The listing builds one solid part. Answer for the finished solid, in the listing's coordinates (mm). A direction names the side the tool comes from. Coordinates: 2 decimals unless noted, no trailing zeros. Order: outer loops, then holes, each group sorted by start corner. A loop starts at its lowest first (then second) coordinate and runs counter-clockwise, first axis right, second up.
from build123d import *

# Parameters (mm, degrees)
SKETCH2_R                            = 3.35
F_40_SERIES_TS40_80LM_650037_1_DEPTH = 300
M8X1_25_TAPPED_HOLE1_AT_2_COUNT      = 2
M8X1_25_TAPPED_HOLE1_AT_2_PITCH      = 40


with BuildPart() as part:
    # Sketch2 → 40 series TS40-80LM-650037(1) (new body)
    with BuildSketch(Plane(origin=(0, 0, 150), x_dir=(-1, 0, 0), z_dir=(0, 0, -1))):
        with BuildLine():
            Line((0, -27.681), (-5.525738531, -27.681))
            Line((-5.525738531, -27.681), (-11.176, -33.331261469))
            Line((-11.176, -33.331261469), (-11.176, -36.6218))
            Line((-11.176, -36.6218), (-7.6835, -36.6218))
            Line((-7.6835, -36.6218), (-7.6835, -35.2248))
            Line((-7.6835, -35.2248), (-4.0488, -35.2248))
            Line((-4.0488, -35.2248), (-4.0488, -40))
            Line((-4.0488, -40), (-17, -40))
            ThreePointArc((-17, -40), (-19.121320344, -39.121320344), (-20, -37))
            Line((-20, -37), (-20, -24.0488))
            Line((-20, -24.0488), (-15.2248, -24.0488))
            Line((-15.2248, -24.0488), (-15.2248, -27.6835))
            Line((-15.2248, -27.6835), (-16.6218, -27.6835))
            Line((-16.6218, -27.6835), (-16.6218, -31.176))
            Line((-16.6218, -31.176), (-13.331261469, -31.176))
            Line((-13.331261469, -31.176), (-7.681, -25.525738531))
            Line((-7.681, -25.525738531), (-7.681, -20))
            Line((-7.681, -20), (-7.681, -14.474261469))
            Line((-7.681, -14.474261469), (-13.331261469, -8.824))
            Line((-13.331261469, -8.824), (-16.6218, -8.824))
            Line((-16.6218, -8.824), (-16.6218, -12.3165))
            Line((-16.6218, -12.3165), (-15.2248, -12.3165))
            Line((-15.2248, -12.3165), (-15.2248, -15.9512))
            Line((-15.2248, -15.9512), (-20, -15.9512))
            Line((-20, -15.9512), (-20, 15.9512))
            Line((-20, 15.9512), (-15.2248, 15.9512))
            Line((-15.2248, 15.9512), (-15.2248, 12.3165))
            Line((-15.2248, 12.3165), (-16.6218, 12.3165))
            Line((-16.6218, 12.3165), (-16.6218, 8.824))
            Line((-16.6218, 8.824), (-13.331261469, 8.824))
            Line((-13.331261469, 8.824), (-7.681, 14.474261469))
            Line((-7.681, 14.474261469), (-7.681, 25.525738531))
            Line((-7.681, 25.525738531), (-13.331261469, 31.176))
            Line((-13.331261469, 31.176), (-16.6218, 31.176))
            Line((-16.6218, 31.176), (-16.6218, 27.6835))
            Line((-16.6218, 27.6835), (-15.2248, 27.6835))
            Line((-15.2248, 27.6835), (-15.2248, 24.0488))
            Line((-15.2248, 24.0488), (-20, 24.0488))
            Line((-20, 24.0488), (-20, 37))
            ThreePointArc((-20, 37), (-19.121320344, 39.121320344), (-17, 40))
            Line((-17, 40), (-4.0488, 40))
            Line((-4.0488, 40), (-4.0488, 35.2248))
            Line((-4.0488, 35.2248), (-7.6835, 35.2248))
            Line((-7.6835, 35.2248), (-7.6835, 36.6218))
            Line((-7.6835, 36.6218), (-11.176, 36.6218))
            Line((-11.176, 36.6218), (-11.176, 33.331261469))
            Line((-11.176, 33.331261469), (-5.525738531, 27.681))
            Line((-5.525738531, 27.681), (0, 27.681))
            Line((0, 27.681), (5.525738531, 27.681))
            Line((5.525738531, 27.681), (11.176, 33.331261469))
            Line((11.176, 33.331261469), (11.176, 36.6218))
            Line((11.176, 36.6218), (7.6835, 36.6218))
            Line((7.6835, 36.6218), (7.6835, 35.2248))
            Line((7.6835, 35.2248), (4.0488, 35.2248))
            Line((4.0488, 35.2248), (4.0488, 40))
            Line((4.0488, 40), (17, 40))
            ThreePointArc((17, 40), (19.121320344, 39.121320344), (20, 37))
            Line((20, 37), (20, 24.0488))
            Line((20, 24.0488), (15.2248, 24.0488))
            Line((15.2248, 24.0488), (15.2248, 27.6835))
            Line((15.2248, 27.6835), (16.6218, 27.6835))
            Line((16.6218, 27.6835), (16.6218, 31.176))
            Line((16.6218, 31.176), (13.331261469, 31.176))
            Line((13.331261469, 31.176), (7.681, 25.525738531))
            Line((7.681, 25.525738531), (7.681, 20))
            Line((7.681, 20), (7.681, 14.474261469))
            Line((7.681, 14.474261469), (13.331261469, 8.824))
            Line((13.331261469, 8.824), (16.6218, 8.824))
            Line((16.6218, 8.824), (16.6218, 12.3165))
            Line((16.6218, 12.3165), (15.2248, 12.3165))
            Line((15.2248, 12.3165), (15.2248, 15.9512))
            Line((15.2248, 15.9512), (20, 15.9512))
            Line((20, 15.9512), (20, -15.9512))
            Line((20, -15.9512), (15.2248, -15.9512))
            Line((15.2248, -15.9512), (15.2248, -12.3165))
            Line((15.2248, -12.3165), (16.6218, -12.3165))
            Line((16.6218, -12.3165), (16.6218, -8.824))
            Line((16.6218, -8.824), (13.331261469, -8.824))
            Line((13.331261469, -8.824), (7.681, -14.474261469))
            Line((7.681, -14.474261469), (7.681, -20))
            Line((7.681, -20), (7.681, -25.525738531))
            Line((7.681, -25.525738531), (13.331261469, -31.176))
            Line((13.331261469, -31.176), (16.6218, -31.176))
            Line((16.6218, -31.176), (16.6218, -27.6835))
            Line((16.6218, -27.6835), (15.2248, -27.6835))
            Line((15.2248, -27.6835), (15.2248, -24.0488))
            Line((15.2248, -24.0488), (20, -24.0488))
            Line((20, -24.0488), (20, -37))
            ThreePointArc((20, -37), (19.121320344, -39.121320344), (17, -40))
            Line((17, -40), (4.0488, -40))
            Line((4.0488, -40), (4.0488, -35.2248))
            Line((4.0488, -35.2248), (7.6835, -35.2248))
            Line((7.6835, -35.2248), (7.6835, -36.6218))
            Line((7.6835, -36.6218), (11.176, -36.6218))
            Line((11.176, -36.6218), (11.176, -33.331261469))
            Line((11.176, -33.331261469), (5.525738531, -27.681))
            Line((5.525738531, -27.681), (0, -27.681))
        make_face()
        with Locations((0, -20)):
            Circle(SKETCH2_R, mode=Mode.SUBTRACT)
        with Locations((0, 20)):
            Circle(SKETCH2_R, mode=Mode.SUBTRACT)
        Polygon((-5.525738531, 12.319), (-17.844738531, 0), (-5.525738531, -12.319), (0, -12.319), (5.525738531, -12.319), (17.844738531, 0), (5.525738531, 12.319), (0, 12.319), align=None, mode=Mode.SUBTRACT)
        with BuildLine():
            Line((12.8372, 38.222), (12.8372, 32.8372))
            Line((12.8372, 32.8372), (18.222, 32.8372))
            Line((18.222, 32.8372), (18.222, 35.428))
            ThreePointArc((18.222, 35.428), (17.403656347, 37.403656347), (15.428, 38.222))
            Line((15.428, 38.222), (12.8372, 38.222))
        make_face(mode=Mode.SUBTRACT)
        with BuildLine():
            Line((12.8372, -32.8372), (18.222, -32.8372))
            Line((18.222, -32.8372), (18.222, -35.428))
            ThreePointArc((18.222, -35.428), (17.403656347, -37.403656347), (15.428, -38.222))
            Line((15.428, -38.222), (12.8372, -38.222))
            Line((12.8372, -38.222), (12.8372, -32.8372))
        make_face(mode=Mode.SUBTRACT)
        with BuildLine():
            Line((-12.8372, -38.222), (-12.8372, -32.8372))
            Line((-12.8372, -32.8372), (-18.222, -32.8372))
            Line((-18.222, -32.8372), (-18.222, -35.428))
            ThreePointArc((-18.222, -35.428), (-17.403656347, -37.403656347), (-15.428, -38.222))
            Line((-15.428, -38.222), (-12.8372, -38.222))
        make_face(mode=Mode.SUBTRACT)
        with BuildLine():
            Line((-18.222, 35.428), (-18.222, 32.8372))
            Line((-18.222, 32.8372), (-12.8372, 32.8372))
            Line((-12.8372, 32.8372), (-12.8372, 38.222))
            Line((-12.8372, 38.222), (-15.428, 38.222))
            ThreePointArc((-15.428, 38.222), (-17.403656347, 37.403656347), (-18.222, 35.428))
        make_face(mode=Mode.SUBTRACT)
    extrude(amount=F_40_SERIES_TS40_80LM_650037_1_DEPTH)

    # Sketch4 → M8x1.25 Tapped Hole1 (revolve, cut)
    with BuildSketch(Plane(origin=(0, -20, 150), x_dir=(0, -1, 0), z_dir=(1, 0, 0))):
        Polygon((0, 0), (0, 32.042926105), (3.4, 30), (3.4, 0), align=None)
    m8x1_25_tapped_hole1 = revolve(axis=Axis((0, -20, 156.35), (0, 0, -1)), mode=Mode.SUBTRACT)

    # M8x1.25 Tapped Hole1 at 2: M8x1.25 Tapped Hole1 ×2
    with Locations(*[(0, i * M8X1_25_TAPPED_HOLE1_AT_2_PITCH, 0) for i in range(1, M8X1_25_TAPPED_HOLE1_AT_2_COUNT)]):
        add(m8x1_25_tapped_hole1, mode=Mode.SUBTRACT)

    # Mirror1: M8x1.25 Tapped Hole1 across plane
    add(m8x1_25_tapped_hole1.mirror(Plane.XY), mode=Mode.SUBTRACT)

    # Mirror1 copy 1 sketch → Mirror1 copy 1 (revolve, cut)
    with BuildSketch(Plane(origin=(0, 20, -150), x_dir=(0, -1, 0), z_dir=(1, 0, 0))):
        Polygon((0, 0), (0, -32.042926105), (3.4, -30), (3.4, 0), align=None)
    revolve(axis=Axis((0, 20, -156.35), (0, 0, -1)), mode=Mode.SUBTRACT)


solid = part.part
(1) Find section B-B on y = -20. Determine the outline of the cut face in (x, z), then the cut area to 3 significant figures.
(2) Given pin 1 Ø1.4 at (y, z) = (38.5, -69) entering from -X; pin 2 Ø5.5 at (x, z) = (-1, 32) entering from +Y, each flat-ended and moving along its own axis, determine where each tip first touches the part or whether it passes through.
(3) Find the intervals of material crossed by probe 1 along Y at (x, z) = (0, 141.25); probe 2 along Y at (x, z) = (0, 26); probe 3 along X at (y, z) = (20, -32.5), in increasing order.
(4) The mould has two halves that part along X. Classify faces 5 (the flat face through (-10.546, 28.39, 2.1)), 6 (the flat face through (-11, -40, 2)), 7 (the flat face through (-20, -30, 2)): pulls with the +X half, pulls with the -X half, needs draft (parallel to the pull), parting line crosses it, or undercut.
(5) A tool of negligible diameter and unlimited length cuts with its end or side. For faces 1 (the flat face through (-10.467, -28.311, 2.1)), 2 (the flat face through (-4.049, 38, 2)), 3 (the flat face through (18, -15.951, 2)), 4 (the flat face through (20, -31, 2)), from which of +Z, -Z, +X, -X, +Y, -Y can it reach the whole face along a straight path? Write none if from no direction.
(6) Find section A-A on x = 0. Count the separate pieces of the cut face and the enclosed holes in it, then the cut area to 3 significant figures.
Resolved:
1. outline: (-7.68, -150) - (-3.4, -150) - (-3.4, -120) - (-3.35, -119.97) - (-3.35, 119.97) - (-3.4, 120) - (-3.4, 150) - (-7.68, 150) - close; (3.35, -119.97) - (3.4, -120) - (3.4, -150) - (7.68, -150) - (7.68, 150) - (3.4, 150) - (3.4, 120) - (3.35, 119.97) - close
1. area: 2,590 mm2
2. pin 1: stops at x = -19.89
2. pin 2: stops at y = 27.68
3. probe 1: y = -27.68 to -23.4, -16.6 to -12.32, 12.32 to 16.6, 23.4 to 27.68
3. probe 2: y = -27.68 to -23.35, -16.65 to -12.32, 12.32 to 16.65, 23.35 to 27.68
3. probe 3: x = -7.68 to -3.35, 3.35 to 7.68
4. face 5: undercut
4. face 6: needs draft
4. face 7: pulls with the -X half
5. face 1: +Z, -Z
5. face 2: +Z, -Z, +Y
5. face 3: +Z, -Z, +X
5. face 4: +Z, -Z, +X, +Y, -Y
6. separate pieces: 4
6. enclosed holes: 0
6. area: 5,190 mm2
